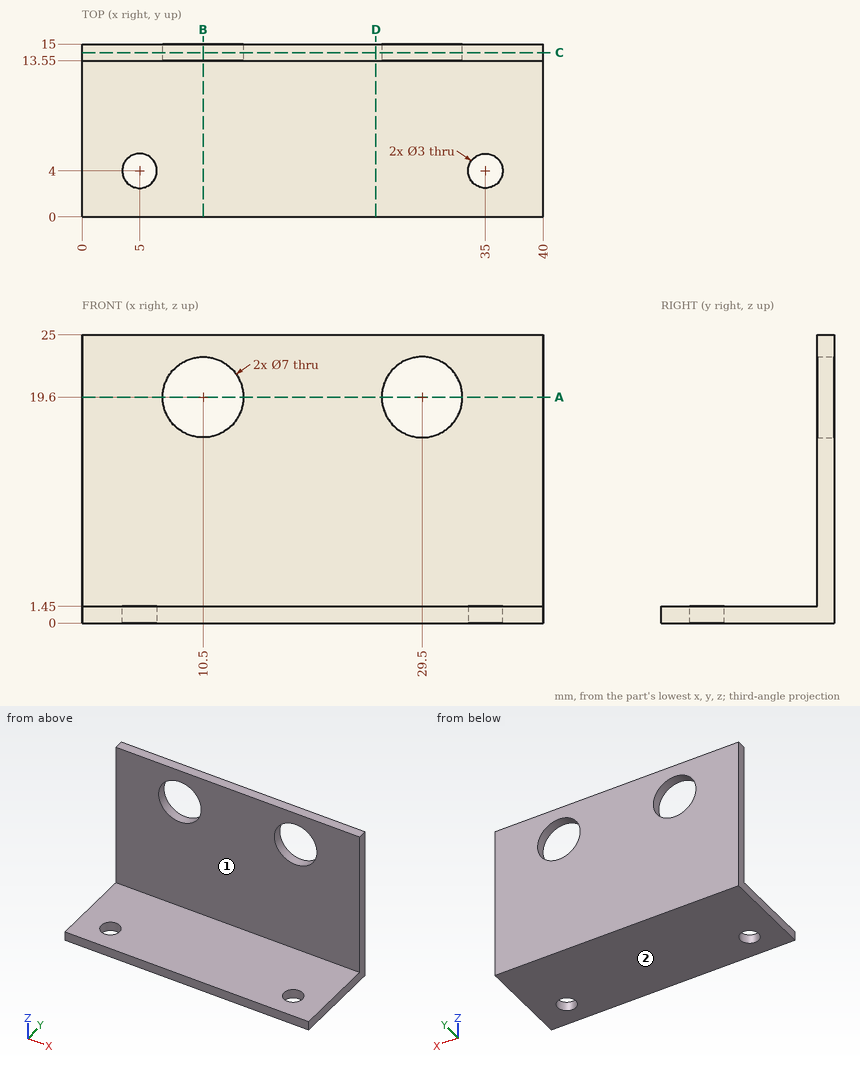
Study the drawing (mm; zero at the part's minimum x, y, z) and answer. A direction names the side the tool comes from. Give positions to 0.01 mm unless a question says otherwise; leave off trailing zeros. Order: outer loops, then holes, each group sorted by start corner. A loop starts at its lowest first (then second) coordinate and runs counter-clockwise, first axis right, second up.
1) Find section C-C on y = 14.25. Write down the section's boundary in (x, z), then the cut area to 3 significant figures.
Reported:
outline: (0, 0) - (40, 0) - (40, 25) - (0, 25) - close; hole circle Ø7 at (10.5, 19.6); hole circle Ø7 at (29.5, 19.6)
area: 923 mm2
2) For the marked faces 1 and 2, determine the directions among +Z, -Z, +X, -X, +Y, -Y from which every point of the face is accessible in a straight line to the end or side of a thin tool.
Reported:
face 1: +Z, +X, -X, -Y
face 2: -Z, +X, -X, +Y, -Y
3) Find section A-A on z = 19.6. Write down the section's boundary in (x, y).
Reported:
outline: (0, 13.55) - (7, 13.55) - (7, 15) - (0, 15) - close; (14, 13.55) - (26, 13.55) - (26, 15) - (14, 15) - close; (33, 13.55) - (40, 13.55) - (40, 15) - (33, 15) - close
4) Find section D-D on x = 25.5. Write down the section's boundary in (y, z), then the cut area to 3 significant figures.
Reported:
outline: (0, 0) - (15, 0) - (15, 25) - (13.55, 25) - (13.55, 1.45) - (0, 1.45) - close
area: 55.9 mm2
5) Consider line 1 along X through (y, z) = (14.6, 19.6); line 2 along Z through (x, y) = (10.5, 14.7); line 3 along Y through (x, z) = (35, 0.6). Determine where each line is inside the solid, lowest interval first.
Reported:
line 1: x = 0 to 7, 14 to 26, 33 to 40
line 2: z = 0 to 16.1, 23.1 to 25
line 3: y = 0 to 2.5, 5.5 to 15
6) Find section B-B on x = 10.5. Write down the section's boundary in (y, z), then the cut area to 3 significant figures.
Reported:
outline: (0, 0) - (15, 0) - (15, 16.1) - (13.55, 16.1) - (13.55, 1.45) - (0, 1.45) - close; (13.55, 23.1) - (15, 23.1) - (15, 25) - (13.55, 25) - close
area: 45.7 mm2
7) Given P1, Ø6, axis at y = 12.5, z = 18.5, coming from the -X side; P2, Ø4, axis at x = 35, y = 4, coming from the +Z side, each flat-ended and moving along its own axis, determine where each tip first touches the part or whether it passes through.
Reported:
P1: stops at x = 0
P2: stops at z = 1.45
